Part model, mm, in its own coordinate system. A direction names the side the tool comes from. Round coordinates to 2 decimals unless told otherwise and drop trailing zeros. Loops run counter-clockwise (first coordinate to the right, second up) from the corner with the lowest first, then second, coordinate; pieces in that order, holes last. Notation, with made-up numbers: (40.5, 35) -> (64.5, 35) arc R20 ccw to (64.5, 48) -> close; hole circle Ø1 at (11, 35). An arc over 180 degrees is marked (long way). Answer as a JSON object with one key per item and string values. Group by question number.
Autodesk Inventor part; units mm, degrees
ref_plane "YZ Plane" through (0, 0, 0) normal (1, 0, 0) x (0, 1, 0)
ref_plane "XZ Plane" through (0, 0, 0) normal (0, 1, 0) x (-1, 0, 0)
ref_plane "XY Plane" through (0, 0, 0) normal (0, 0, 1) x (1, 0, 0)
sketch "スケッチ1" plane through (0, 0, 0) normal (0, 0, 1) x (1, 0, 0)
  line L0 (7.5, -7.5) -> (-7.5, -7.5)
  line L1 (-7.5, -7.5) -> (-7.5, 7.5)
  line L2 (-7.5, 7.5) -> (7.5, 7.5)
  line L3 (7.5, 7.5) -> (7.5, -7.5)
  line L4 (7.5, -7.5) -> (-7.5, 7.5) construction
  line L5 (-7.5, -7.5) -> (7.5, 7.5) construction
  point P0 (0, 0)
  dimension "d0" = 15
  dimension "d1" = 15
extrude "押し出し1" add sketch "スケッチ1" along normal blind 280
shell "シェル1" thickness 1 removed faces 2 at (2.5, -2.5, 0) at (2.5, -2.5, 280)
sketch "スケッチ2" plane through (-7.5, 7.5, 0) normal (0, 1, 0) x (1, 0, 0)
  line L0 (7.5, -172.043) -> (7.5, -107.957) construction
  line L1 (15, -280) -> (0, -280)
  line L2 (0, 0) -> (0, -280)
  line L3 (0, -140) -> (7.5, -140) construction
  point P0 (7.5, 0)
  point P1 (7.5, -280)
  point P2 (7.5, -272)
  point P3 (7.5, -8)
  dimension "d5" = 64.086
  dimension "d29" = 264
hole "穴1" at (0, 7.5, 172.043) at (0, 7.5, 107.957) at (0, 7.5, 272) at (0, 7.5, 8) direction (0, -1, 0) diameter 3.2 end through all
sketch "スケッチ3" plane through (-7.5, -7.5, 0) normal (-1, 0, 0) x (0, 0, 1)
  line L0 (20, 7.5) -> (260, 7.5)
  line L1 (0, 15) -> (280, 15)
  line L2 (280, 15) -> (280, 0)
  point P0 (0, 7.5)
  point P1 (140, 7.5)
  point P2 (140, 15)
  point P3 (280, 7.5)
  dimension "d13" = 240
hole "穴2" at (-7.5, 0, 260) at (-7.5, 0, 20) direction (1, 0, 0) diameter 5.2 depth 1 tip angle 118
sketch "スケッチ4" plane through (7.5, -7.5, 0) normal (1, 0, 0) x (0, 0, -1)
  circle A0 centre (-260, 7.5) radius 2.6
  circle A1 centre (-20, 7.5) radius 2.6
  line L0 (0, 0) -> (0, 15)
  line L1 (0, 0) -> (-280, 0)
  line L2 (-280, 15) -> (-280, 0)
  line L3 (0, 15) -> (-280, 15)
  point P0 (0, 7.5)
hole "穴3" at (7.5, 0, 20) at (7.5, 0, 260) direction (-1, 0, 0) diameter 10 depth 1 tip angle 118
properties part number "BaseSlideSTOPPERsq"
Item 1: Two-plate mould, pull along Y, no slides. Class faces 4 (the face through (0, 7.5, 138)), 5 (the face through (-6.99, -0.78, 22.48)), 6 (the face through (-7, 0, 280)): pulls with the +Y half, pulls with the -Y half, needs draft (parallel to the pull), parting line crosses it, or undercut.
Item 2: Band-saw the part on A-A, the plane y = 0. List the corners of the cut face in (x, z).
Item 3: Drill centre lines: line 1 (Z direction, x = 7.3, y = 0); line 2 (Z direction, x = 0, y = -7.2); line 3 (Z direction, x = -6.7, y = 0). Where is each one in solid material? Low to high.
Item 4: Band-saw the part on C-C, the plane z = 191.5. List the corners of the cut face in (x, y).
Item 5: Band-saw the part on B-B, the plane z = 260. List the corners of the cut face in (x, y), plus the area to 3 significant figures.
Item 6: Which spindle directions (+Z, -Z, +X, -X, +Y, -Y) get a long thin tool onto all of the face, cutting with end or side? Do faces 1 (the face through (6.5, 0, 138)), 2 (the face through (0, -7.5, 138)), 3 (the face through (6.99, -1.5, 255.23)). Say none if no direction does.
Entries:
{
 "1": {"face 4": "pulls with the +Y half", "face 5": "undercut", "face 6": "needs draft"},
 "2": {"outline": "(-7.5, 0) -> (-6.5, 0) -> (-6.5, 17.4) -> (-7.5, 17.4) -> close; (-7.5, 22.6) -> (-6.5, 22.6) -> (-6.5, 257.4) -> (-7.5, 257.4) -> close; (-7.5, 262.6) -> (-6.5, 262.6) -> (-6.5, 280) -> (-7.5, 280) -> close; (6.5, 0) -> (7.5, 0) -> (7.5, 15) -> (6.5, 15) -> close; (6.5, 25) -> (7.5, 25) -> (7.5, 255) -> (6.5, 255) -> close; (6.5, 265) -> (7.5, 265) -> (7.5, 280) -> (6.5, 280) -> close"},
 "3": {"line 1": "0 to 15, 25 to 255, 265 to 280", "line 2": "0 to 6.4, 9.6 to 106.36, 109.56 to 170.44, 173.64 to 270.4, 273.6 to 280", "line 3": "0 to 17.4, 22.6 to 257.4, 262.6 to 280"},
 "4": {"outline": "(-7.5, -7.5) -> (7.5, -7.5) -> (7.5, 7.5) -> (-7.5, 7.5) -> close; hole (-6.5, -6.5) -> (6.5, -6.5) -> (6.5, 6.5) -> (-6.5, 6.5) -> close"},
 "5": {"outline": "(-7.5, -7.5) -> (7.5, -7.5) -> (7.5, -5) -> (6.5, -5) -> (6.5, -6.5) -> (-6.5, -6.5) -> (-6.5, -2.6) -> (-7.5, -2.6) -> close; (-7.5, 2.6) -> (-6.5, 2.6) -> (-6.5, 6.5) -> (6.5, 6.5) -> (6.5, 5) -> (7.5, 5) -> (7.5, 7.5) -> (-7.5, 7.5) -> close", "area": "40.8 mm²"},
 "6": {"face 1": "+Z, -Z", "face 2": "+Z, -Z, +X, -X, -Y", "face 3": "+X"}
}
